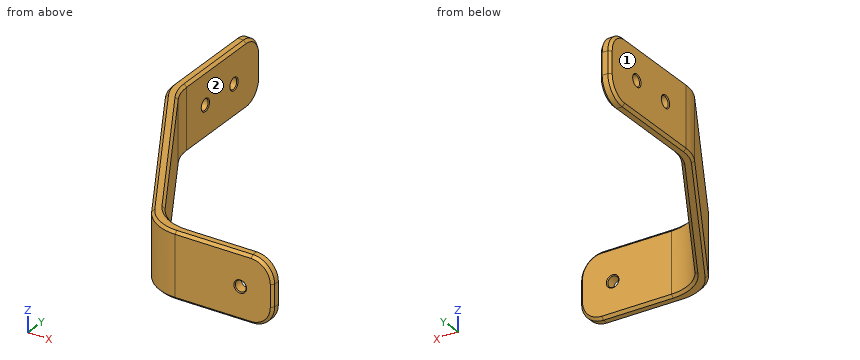
```python
from build123d import *

# Parameters (mm, degrees)
SKETCH2_W                    = 3.175
SKETCH2_H                    = 19.05
F_1_8_0_125_DIAMETER_HOLE1_D = 3.175
F_1_8_0_125_DIAMETER_HOLE2_D = 3.175
FILLET1_R                    = 12.7
FILLET2_R                    = 6.35
CHAMFER3_SIZE                = 0.762
CHAMFER2_SIZE                = 0.254


with BuildPart() as part:
    # Sweep1: sweep along a path in Sketch1
    with BuildLine(Plane.XY) as sweep1_path:
        Line((0, 0), (0, -36.5125))
        Line((0, -36.5125), (33.61082832, -94.728162334))
        Line((33.61082832, -94.728162334), (68.53582832, -94.728162334))
    # Sketch2 → Sweep1 (sweep)
    with BuildSketch(Plane(origin=(0, 0, 0), x_dir=(1, 0, 0), z_dir=(0, 1, 0))):
        Rectangle(SKETCH2_W, SKETCH2_H)
    sweep(path=sweep1_path.line, transition=Transition.RIGHT)

    # 1/8 (0.125) Diameter Hole1 (through all)
    with Locations(Plane(origin=(1.5875, 0, 0), x_dir=(0, 0, -1), z_dir=(1, 0, 0))):
        with Locations((0, -11.693565329), (0, -24.393565329)):
            Hole(F_1_8_0_125_DIAMETER_HOLE1_D / 2)

    # 1/8 (0.125) Diameter Hole2 (through all)
    with Locations(Plane(origin=(0, -93.140662334, 0), x_dir=(1, 0, 0), z_dir=(0, 1, 0))):
        with Locations((59.01082832, 0)):
            Hole(F_1_8_0_125_DIAMETER_HOLE2_D / 2)

    # Fillet1
    fillet1_edges = [part.edges().sort_by_distance(p)[0] for p in [
        (1.5875, -36.087130657, 0),
        (-1.5875, -36.937869343, 0),
        (32.694284767, -96.315662334, 0),
        (34.527371872, -93.140662334, 0),
    ]]
    fillet(fillet1_edges, radius=FILLET1_R)

    # Fillet2
    fillet2_edges = [part.edges().sort_by_distance(p)[0] for p in [
        (0, 0, -9.525),
        (0, 0, 9.525),
        (68.53582832, -94.728162334, -9.525),
        (68.53582832, -94.728162334, 9.525),
    ]]
    fillet(fillet2_edges, radius=FILLET2_R)

    # Chamfer3
    chamfer3_edges = [part.edges().sort_by_distance(p)[0] for p in [
        (68.53582832, -96.315662334, 0),
        (66.67595638, -96.315662334, 7.665128061),
        (66.67595638, -96.315662334, -7.665128061),
        (68.53582832, -93.140662334, 0),
        (66.67595638, -93.140662334, 7.665128061),
        (66.67595638, -93.140662334, -7.665128061),
        (1.5875, 0, 0),
        (-1.5875, 0, 0),
        (-1.5875, -19.9424573, -9.525),
        (-1.5875, -19.9424573, 9.525),
        (-1.5875, -1.859871939, 7.665128061),
        (-1.5875, -1.859871939, -7.665128061),
        (1.5875, -19.517087957, -9.525),
        (1.5875, -19.517087957, 9.525),
        (1.5875, -1.859871939, 7.665128061),
        (1.5875, -1.859871939, -7.665128061),
        (51.106230753, -96.315662334, -9.525),
        (51.106230753, -96.315662334, 9.525),
        (52.022774305, -93.140662334, -9.525),
        (33.676633186, -94.614184962, -9.525),
        (14.571043965, -64.925288467, -9.525),
        (17.075087517, -62.912419124, -9.525),
        (-1.154757994, -36.821916472, -9.525),
        (33.676633186, -94.614184962, -9.525),
        (14.571043965, -64.925288467, 9.525),
        (17.075087517, -62.912419124, 9.525),
        (-1.154757994, -36.821916472, 9.525),
        (33.676633186, -94.614184962, 9.525),
        (52.022774305, -93.140662334, 9.525),
        (33.676633186, -94.614184962, 9.525),
        (-1.154757994, -36.821916472, -9.525),
        (-1.154757994, -36.821916472, 9.525),
        (35.509720291, -91.439184962, 9.525),
        (35.509720291, -91.439184962, 9.525),
        (35.509720291, -91.439184962, -9.525),
        (35.509720291, -91.439184962, -9.525),
        (2.020242006, -35.971177786, 9.525),
        (2.020242006, -35.971177786, 9.525),
        (2.020242006, -35.971177786, -9.525),
        (2.020242006, -35.971177786, -9.525),
    ]]
    chamfer(chamfer3_edges, length=CHAMFER3_SIZE)

    # Chamfer2
    chamfer2_edges = [part.edges().sort_by_distance(p)[0] for p in [
        (1.5875, -24.393565329, -1.5875),
        (-1.5875, -24.393565329, -1.5875),
        (1.5875, -11.693565329, -1.5875),
        (-1.5875, -11.693565329, -1.5875),
        (60.59832832, -93.140662334, 0),
        (60.59832832, -96.315662334, 0),
    ]]
    chamfer(chamfer2_edges, length=CHAMFER2_SIZE)


solid = part.part
```
Model file for the job. Use its own axes, mm. Face numbers are marked on the shaded views. A direction names the side the tool comes from. Coordinates: 2 decimals unless noted, no trailing zeros. Write each loop counter-clockwise with the first axis right and the second up, starting at its lowest first coordinate (ties: lowest second). Pieces come first, ordered by that corner, then holes. Notation, with made-up numbers: (29, -22.5) - (66, -22.5) arc R22 ccw to (66, 14.5) - close; hole circle Ø6 at (2.25, 70). An arc over 180 degrees is marked (long way). One line per item, written item: value. Start each with the question number.
1. Slice it at A-A (y = -8.5). Write the cut outline in (x, z) (1 decimal), plus the area to 3 significant figures.
2. Flat gauge pins, fed straight in: pin 1 (10 mm diameter, centred on y = -77, z = -3, fed in from +X); pin 2 (5.5 mm diameter, centred on x = 58, z = 0, fed in from +Y); pin 3 (8 mm diameter, centred on y = -13, z = 5, fed in from +X); pin 4 (3 mm diameter, centred on y = -11.69, z = 0, fed in from -X). Where does each tip first touch, or does it go through?
3. Tool access for the marked faces 1 and 2: list every direction of +Z, -Z, +X, -X, +Y, -Y with a clear straight run to the whole face (end or side of a thin tool).
4. Probe line 1 (Y direction, x = -0.05, z = 0); line 2 (Y direction, x = 0.5, z = 0); line 3 (X direction, y = -4.5, z = 2.25). List the from-to ranges inside material, lowest first. Write a range as from..to.
5. Slice it at B-B (x = 53). Write the cut outline in (y, z) (3 decimals), plus the area to 3 significant figures.
Answers below:
1. outline: (-1.6, -8.8) - (-0.8, -9.5) - (0.8, -9.5) - (1.6, -8.8) - (1.6, 8.8) - (0.8, 9.5) - (-0.8, 9.5) - (-1.6, 8.8) - close
1. area: 59.3 mm^2
2. pin 1: stops at x = 28.1
2. pin 2: stops at y = -93.14
2. pin 3: stops at x = 1.59
2. pin 4: passes through
3. face 1: +Z, -Z, -X, +Y, -Y
3. face 2: +Z, -Z, +X, +Y
4. line 1: y = -39.59..-25.98, -22.81..-13.28, -10.11..0
4. line 2: y = -40.55..-25.98, -22.81..-13.28, -10.11..0
4. line 3: x = -1.59..1.59
5. outline: (-96.316, -8.763) - (-95.554, -9.525) - (-93.903, -9.525) - (-93.141, -8.763) - (-93.141, 8.763) - (-93.903, 9.525) - (-95.554, 9.525) - (-96.316, 8.763) - close
5. area: 59.3 mm^2
